Verification items for the finished model (mm, model axes). A direction names the side the tool comes from. Give positions to 0.01 mm unless a question says otherwise; leave off trailing zeros. Loops run counter-clockwise (first coordinate to the right, second up) from the corner with the lowest first, then second, coordinate; pieces in that order, holes last. Notation, with made-up numbers: (4, -6.75) -> (61, -6.75) arc R21 cw to (61, 14.25) -> close; hole circle Ø7 at (66.25, 54.25). An arc over 180 degrees is marked (long way). Answer in a Markdown table with one row per item. Add a question column.
Q1. Material ranges on probe 1 along X at (y, z) = (24, 4.5); probe 2 along Y at (x, z) = (9, 25); probe 3 along X at (y, z) = (6, 31), recorded low to high.
Q2. Set-up check for faces 1 (the face through (-1.5, 12, 9)), 2 (the face through (0, 12, 20)), 3 (the face through (-7.43, 12.44, 27.6)), 4 (the face through (-4, 16.5, 31)): record each of +Z, -Z, +X, -X, +Y, -Y from which the full face is reachable in a straight line by a thin tool's end or side.
Q3. Section check B-B on y = 20.75. Enter the section's corners in (x, z), and give its area (3 significant figures).
Q4. Section check D-D on x = 47.6. Enter the section's corners in (y, z), and give its area (3 significant figures).
Q5. Section check A-A on x = 32.5. Enter the section's corners in (y, z), and give its area (3 significant figures).
Q6. Section check C-C on x = 3.5. Enter the section's corners in (y, z).
Q7. Gauge pin test, flat ends, axial feed: P1, Ø4.5, axis at x = 32.5, z = 20, coming from the -Y side; P2, Ø0.5, axis at x = -5.5, y = 15.5, coming from the +Z side; P3, Ø2, axis at x = -3.5, z = 9, coming from the -Y side; P4, Ø3, axis at y = 17.5, z = 15.5, coming from the -X side. Record the tip position at first contact, or that the pin passes through.
Q8. Release check for a two-part mould opening along X. For faces 5 (the face through (30, 24, 40)), 6 (the face through (-0.35, 7.63, 9.13)), 7 (the face through (-4, 15, 31)) record: pulls with the +X half, pulls with the -X half, needs draft (parallel to the pull), parting line crosses it, or undercut.
```python
from build123d import *

# Parameters (mm, degrees)
SKETCH1_W           = 65
SKETCH1_H           = 40
BOSS_EXTRUDE1_DEPTH = 25
SKETCH8_W           = 61
SKETCH8_H           = 21
CUT_EXTRUDE1_DEPTH  = 40
SKETCH9_R           = 2.5
CUT_EXTRUDE2_DEPTH  = 30
SKETCH10_R          = 3.881431072
CUT_EXTRUDE3_DEPTH  = 26
SKETCH11_W          = 8
SKETCH11_H          = 8
BOSS_EXTRUDE2_DEPTH = 8
SKETCH12_W          = 5
SKETCH12_H          = 5
CUT_EXTRUDE4_DEPTH  = 52
FILLET1_R           = 2
FILLET2_START       = 6.4999999
FILLET2_DEPTH       = 12.0000001
FILLET2_START_2     = 7.897261538
FILLET2_2_DEPTH     = 2.102738462
FILLET2_START_3     = 15
FILLET2_3_DEPTH     = 2.089446154
FILLET2_START_4     = -1
FILLET2_4_DEPTH     = 42
FILLET3_START       = 5
FILLET3_DEPTH       = 30
FILLET3_START_2     = 8
FILLET3_2_DEPTH     = 9


with BuildPart() as part:
    # Sketch1 → Boss-Extrude1 (new body)
    with BuildSketch(Plane(origin=(0, 0, 0), x_dir=(1, 0, 0), z_dir=(0, 1, 0))):
        with Locations((32.5, -20)):
            Rectangle(SKETCH1_W, SKETCH1_H)
    extrude(amount=BOSS_EXTRUDE1_DEPTH)

    # Sketch8 → Cut-Extrude1 (cut)
    with BuildSketch(Plane(origin=(0, 0, 0), x_dir=(-1, 0, 0), z_dir=(0, 0, -1))):
        with Locations((-32.5, 12.5)):
            Rectangle(SKETCH8_W, SKETCH8_H)
    extrude(amount=-CUT_EXTRUDE1_DEPTH, mode=Mode.SUBTRACT)

    # Sketch9 → Cut-Extrude2 (cut)
    with BuildSketch(Plane(origin=(0, 25, 0), x_dir=(1, 0, 0), z_dir=(0, 1, 0))):
        with Locations(Location((32.5, -20, 0), (0, 0, 270))):
            Circle(SKETCH9_R)
    extrude(amount=-CUT_EXTRUDE2_DEPTH, mode=Mode.SUBTRACT)

    # Sketch10 → Cut-Extrude3 (cut)
    with BuildSketch(Plane.XZ):
        with Locations(Location((17.4, 4.5, 0), (0, 0, 90))):
            Circle(SKETCH10_R)
        with Locations(Location((47.6, 4.5, 0), (0, 0, 90))):
            Circle(SKETCH10_R)
    extrude(amount=-CUT_EXTRUDE3_DEPTH, mode=Mode.SUBTRACT)

    # Sketch11 → Boss-Extrude2 (add)
    with BuildSketch(Plane.ZY):
        with Locations((9, 12.5)):
            Rectangle(SKETCH11_W, SKETCH11_H)
        with Locations((31, 12.5)):
            Rectangle(SKETCH11_W, SKETCH11_H)
    extrude(amount=BOSS_EXTRUDE2_DEPTH)

    # Sketch12 → Cut-Extrude4 (cut)
    with BuildSketch(Plane(origin=(0, 0, 5), x_dir=(-1, 0, 0), z_dir=(0, 0, -1))):
        with Locations((4, 12.5)):
            Rectangle(SKETCH12_W, SKETCH12_H)
    extrude(amount=-CUT_EXTRUDE4_DEPTH, mode=Mode.SUBTRACT)

    # Fillet1
    fillet1_edges = [part.edges().sort_by_distance(p)[0] for p in [
        (0, 8.5, 9),
        (0, 16.5, 9),
        (0, 8.5, 31),
        (0, 16.5, 31),
    ]]
    fillet(fillet1_edges, radius=FILLET1_R)

    # Fillet2: read off the stored shape, not the designer's step
    # Fillet2 outline → Fillet2 (add)
    with BuildSketch(Plane(origin=(0, 0, 0), x_dir=(1, 0, 0), z_dir=(0, 1, 0)).offset(FILLET2_START)):
        with BuildLine():
            ThreePointArc((-1.5, -14.429285786), (-0.390227771, -16.063508327), (0, -18))
            Line((0, -18), (0, -13))
            Line((0, -13), (-1.5, -13))
            Line((-1.5, -13), (-1.5, -14.429285786))
        make_face()
        with BuildLine():
            Line((-1.5, -35), (-1.5, -36.429285786))
            ThreePointArc((-1.5, -36.429285786), (-0.390227771, -38.063508327), (0, -40))
            Line((0, -40), (0, -35))
            Line((0, -35), (-1.5, -35))
        make_face()
        with BuildLine():
            Line((-1.5, -25.570714214), (-1.5, -27))
            Line((-1.5, -27), (0, -27))
            Line((0, -27), (0, -22))
            ThreePointArc((0, -22), (-0.390227771, -23.936491673), (-1.5, -25.570714214))
        make_face()
        with BuildLine():
            Line((-1.5, -5), (0, -5))
            Line((0, -5), (0, 0))
            ThreePointArc((0, 0), (-0.390227771, -1.936491673), (-1.5, -3.570714214))
            Line((-1.5, -3.570714214), (-1.5, -5))
        make_face()
    extrude(amount=FILLET2_DEPTH)

    # Fillet2 2 outline → Fillet2 2 (add)
    with BuildSketch(Plane(origin=(0, 0, 0), x_dir=(1, 0, 0), z_dir=(0, 1, 0)).offset(FILLET2_START_2)):
        with BuildLine():
            ThreePointArc((-5, -35), (-3.109705191, -35.371092404), (-1.5, -36.429285786))
            Line((-1.5, -36.429285786), (-1.5, -35))
            Line((-1.5, -35), (-5, -35))
        make_face()
        with BuildLine():
            Line((-5, -27), (-1.5, -27))
            Line((-1.5, -27), (-1.5, -25.570714214))
            ThreePointArc((-1.5, -25.570714214), (-3.109705191, -26.628907596), (-5, -27))
        make_face()
        with BuildLine():
            ThreePointArc((-5, -13), (-3.109705191, -13.371092404), (-1.5, -14.429285786))
            Line((-1.5, -14.429285786), (-1.5, -13))
            Line((-1.5, -13), (-5, -13))
        make_face()
        with BuildLine():
            Line((-5, -5), (-1.5, -5))
            Line((-1.5, -5), (-1.5, -3.570714214))
            ThreePointArc((-1.5, -3.570714214), (-3.109705191, -4.628907596), (-5, -5))
        make_face()
    extrude(amount=FILLET2_2_DEPTH)

    # Fillet2 3 outline → Fillet2 3 (add)
    with BuildSketch(Plane(origin=(0, 0, 0), x_dir=(1, 0, 0), z_dir=(0, 1, 0)).offset(FILLET2_START_3)):
        with BuildLine():
            ThreePointArc((-5, -35), (-3.109705191, -35.371092404), (-1.5, -36.429285786))
            Line((-1.5, -36.429285786), (-1.5, -35))
            Line((-1.5, -35), (-5, -35))
        make_face()
        with BuildLine():
            Line((-5, -27), (-1.5, -27))
            Line((-1.5, -27), (-1.5, -25.570714214))
            ThreePointArc((-1.5, -25.570714214), (-3.109705191, -26.628907596), (-5, -27))
        make_face()
        with BuildLine():
            ThreePointArc((-5, -13), (-3.109705191, -13.371092404), (-1.5, -14.429285786))
            Line((-1.5, -14.429285786), (-1.5, -13))
            Line((-1.5, -13), (-5, -13))
        make_face()
        with BuildLine():
            Line((-5, -5), (-1.5, -5))
            Line((-1.5, -5), (-1.5, -3.570714214))
            ThreePointArc((-1.5, -3.570714214), (-3.109705191, -4.628907596), (-5, -5))
        make_face()
    extrude(amount=FILLET2_3_DEPTH)

    # Fillet2 4 outline → Fillet2 4 (cut)
    with BuildSketch(Plane.XY.offset(FILLET2_START_4)):
        with BuildLine():
            Line((-5, 16.5), (-2, 16.5))
            ThreePointArc((-2, 16.5), (-0.585786438, 17.085786438), (0, 18.5))
            Line((0, 18.5), (-1.5, 18.5))
            Line((-1.5, 18.5), (-1.5, 17.089446154))
            Line((-1.5, 17.089446154), (-5, 17.089446154))
            Line((-5, 17.089446154), (-5, 16.5))
        make_face()
        with BuildLine():
            Line((-5, 7.897261538), (-1.5, 7.897261538))
            Line((-1.5, 7.897261538), (-1.5, 6.4999999))
            Line((-1.5, 6.4999999), (0, 6.49999995))
            ThreePointArc((0, 6.49999995), (-0.58578642, 7.914213545), (-2, 8.5))
            Line((-2, 8.5), (-5, 8.5))
            Line((-5, 8.5), (-5, 7.897261538))
        make_face()
    extrude(amount=FILLET2_4_DEPTH, mode=Mode.SUBTRACT)

    # Fillet3: read off the stored shape, not the designer's step
    # Fillet3 outline → Fillet3 (cut)
    with BuildSketch(Plane.XY.offset(FILLET3_START)):
        with BuildLine():
            Line((-8, 8.5), (-6, 8.5))
            ThreePointArc((-6, 8.5), (-7.414213562, 9.085786438), (-8, 10.5))
            Line((-8, 10.5), (-8, 8.5))
        make_face()
        with BuildLine():
            Line((-8, 16.5), (-8, 14.5))
            ThreePointArc((-8, 14.5), (-7.414213562, 15.914213562), (-6, 16.5))
            Line((-6, 16.5), (-8, 16.5))
        make_face()
    extrude(amount=FILLET3_DEPTH, mode=Mode.SUBTRACT)

    # Fillet3 2 outline → Fillet3 2 (cut)
    with BuildSketch(Plane(origin=(0, 0, 0), x_dir=(1, 0, 0), z_dir=(0, 1, 0)).offset(FILLET3_START_2)):
        with BuildLine():
            Line((-8, -35), (-6, -35))
            ThreePointArc((-6, -35), (-7.414213562, -34.414213562), (-8, -33))
            Line((-8, -33), (-8, -35))
        make_face()
        with BuildLine():
            Line((-8, -27), (-8, -29))
            ThreePointArc((-8, -29), (-7.414213562, -27.585786438), (-6, -27))
            Line((-6, -27), (-8, -27))
        make_face()
        with BuildLine():
            Line((-8, -13), (-6, -13))
            ThreePointArc((-6, -13), (-7.414213562, -12.414213562), (-8, -11))
            Line((-8, -11), (-8, -13))
        make_face()
        with BuildLine():
            Line((-8, -5), (-8, -7))
            ThreePointArc((-8, -7), (-7.414213562, -5.585786438), (-6, -5))
            Line((-6, -5), (-8, -5))
        make_face()
    extrude(amount=FILLET3_2_DEPTH, mode=Mode.SUBTRACT)


solid = part.part
```
Taken from the geometry:
| question | item | result |
|---|---|---|
| 1 | probe 1 | x = 0 to 13.52, 21.28 to 43.72, 51.48 to 65 |
| 1 | probe 2 | y = 0 to 2, 23 to 25 |
| 1 | probe 3 | x = 0 to 2, 63 to 65 |
| 2 | face 1 | +Z, -Z |
| 2 | face 2 | -X |
| 2 | face 3 | -X, +Y, -Y |
| 2 | face 4 | +Z, -Z, -X, +Y |
| 3 | outline | (0, 0) -> (2, 0) -> (2, 40) -> (0, 40) -> close; (63, 0) -> (65, 0) -> (65, 40) -> (63, 40) -> close |
| 3 | area | 160 mm² |
| 4 | outline | (0, 0) -> (2, 0) -> (2, 0.62) -> (0, 0.62) -> close; (0, 8.38) -> (2, 8.38) -> (2, 40) -> (0, 40) -> close; (23, 0) -> (25, 0) -> (25, 0.62) -> (23, 0.62) -> close; (23, 8.38) -> (25, 8.38) -> (25, 40) -> (23, 40) -> close |
| 4 | area | 129 mm² |
| 5 | outline | (0, 0) -> (2, 0) -> (2, 17.5) -> (0, 17.5) -> close; (0, 22.5) -> (2, 22.5) -> (2, 40) -> (0, 40) -> close; (23, 0) -> (25, 0) -> (25, 17.5) -> (23, 17.5) -> close; (23, 22.5) -> (25, 22.5) -> (25, 40) -> (23, 40) -> close |
| 5 | area | 140 mm² |
| 6 | outline | (0, 0) -> (2, 0) -> (2, 40) -> (0, 40) -> close; (23, 0) -> (25, 0) -> (25, 40) -> (23, 40) -> close |
| 7 | P1 | passes through |
| 7 | P2 | stops at z = 35 |
| 7 | P3 | stops at y = 8.5 |
| 7 | P4 | stops at x = -1.59 |
| 8 | face 5 | needs draft |
| 8 | face 6 | pulls with the -X half |
| 8 | face 7 | undercut |
